from build123d import *

# Parameters (mm, degrees)
PAD011_DEPTH    = 1.2
PAD012_DEPTH    = 15.6
PAD013_DEPTH    = 1.2
PAD014_DEPTH    = 1.6
PAD015_DEPTH    = 1.6
CHAMFER004_SIZE = 1
FILLET002_R     = 1


with BuildPart() as part:
    # Sketch018 → Pad011 (new body)
    with BuildSketch(Plane.XY):
        with BuildLine():
            ThreePointArc((-94.2875364362, 7.682478298), (-94.6, 0), (-94.2875364362, -7.682478298))
            Line((-94.2875364362, -7.682478298), (-82.6504571335, -7.6824782979))
            Line((-82.6504571335, 7.682478298), (-82.6504571335, -7.6824782979))
            Line((-94.2875364362, 7.682478298), (-82.6504571335, 7.682478298))
        make_face()
    extrude(amount=PAD011_DEPTH)

    # Sketch019 → Pad012 (join)
    with BuildSketch(Plane.XY.offset(1.2)):
        with BuildLine():
            ThreePointArc((-94.2875364362, 7.682478298), (-94.6, 0), (-94.2875364362, -7.682478298))
            Line((-93.0835083525, -7.682478298), (-94.2875364362, -7.682478298))
            ThreePointArc((-93.0835083525, 7.682478298), (-93.4, 0), (-93.0835083525, -7.682478298))
            Line((-94.2875364362, 7.682478298), (-93.0835083525, 7.682478298))
        make_face()
    extrude(amount=PAD012_DEPTH)

    # Sketch020 → Pad013 (join)
    with BuildSketch(Plane.XY.offset(16.8)):
        with BuildLine():
            ThreePointArc((-94.2875364362, 7.682478298), (-94.6, 0), (-94.2875364362, -7.682478298))
            Line((-94.2875364362, -7.682478298), (-82.6504571335, -7.682478298))
            Line((-82.6504571335, 7.682478298), (-82.6504571335, -7.682478298))
            Line((-94.2875364362, 7.682478298), (-82.6504571335, 7.682478298))
        make_face()
    extrude(amount=PAD013_DEPTH)

    # Sketch021 → Pad014 (join)
    with BuildSketch(Plane.XY.offset(1.2)):
        with BuildLine():
            ThreePointArc((-84.2504571335, 7.682478298), (-84.6, 0), (-84.2504571335, -7.682478298))
            Line((-82.6504571335, -7.682478298), (-84.2504571335, -7.682478298))
            Line((-82.6504571335, 7.682478298), (-82.6504571335, -7.682478298))
            Line((-84.2504571335, 7.682478298), (-82.6504571335, 7.682478298))
        make_face()
    extrude(amount=PAD014_DEPTH)

    # Sketch022 → Pad015 (join)
    with BuildSketch(Plane.XY.offset(16.8)):
        with BuildLine():
            ThreePointArc((-84.2504571335, 7.682478298), (-84.6, 0), (-84.2504571335, -7.682478298))
            Line((-82.6504571335, -7.682478298), (-84.2504571335, -7.682478298))
            Line((-82.6504571335, 7.682478298), (-82.6504571335, -7.682478298))
            Line((-84.2504571335, 7.682478298), (-82.6504571335, 7.682478298))
        make_face()
    extrude(amount=-PAD015_DEPTH)

    # Chamfer004
    chamfer004_edges = [part.edges().sort_by_distance(p)[0] for p in [
        (-82.650457, 0, 2.8),
        (-82.650457, 0, 15.2),
    ]]
    chamfer(chamfer004_edges, length=CHAMFER004_SIZE)

    # Fillet002
    fillet002_edges = [part.edges().sort_by_distance(p)[0] for p in [
        (-94.6, 0, 18),
        (-94.6, 0, 0),
        (-82.650457, 0, 18),
        (-82.650457, 0, 0),
        (-83.950457, -7.682478, 2.8),
        (-83.950457, 7.682478, 2.8),
        (-83.950457, 7.682478, 15.2),
        (-83.950457, -7.682478, 15.2),
    ]]
    fillet(fillet002_edges, radius=FILLET002_R)


with BuildPart() as part_1:
    # Body005 placement: moved
    add(part.part.moved(Location((0, 0, -1.4))))


solid = part_1.part
Geometry: final body of the model. Coordinates: model frame, mm. A direction names the side the tool comes from. Round coordinates to 2 decimals unless told otherwise and drop trailing zeros. Loops run counter-clockwise (first coordinate to the right, second up) from the corner with the lowest first, then second, coordinate; pieces in that order, holes last. Notation, with made-up numbers: M 4.5,22.5 L 42.5,22.5 A11 ccw 42.5,40.5 Z; hole C 81.25,1.5 d6. An arc over 180 degrees is marked long. Put each result on its own line as item: value. Start each with the question number.
(1) Draft query along Z for faces 1 (the face through (-82.65, 0, 0)), 2 (the face through (-89, 0, 16.6)), 3 (the face through (-83.16, 0.11, 0.91)), 4 (the face through (-89, 0, -0.2)). Return one class per face: +Z half, -Z half, draft (parallel to the pull), parting line (faces both ways), or undercut.
(2) Contact query for flat-ended pins moving along their axis: pin 1 Ø1 at (y, z) = (4, 5.5) entering from +X; pin 2 Ø1 at (y, z) = (3.5, 4) entering from -X; pin 3 Ø2 at (y, z) = (5, 9.5) entering from -X. Output: stop coordinate, or through.
(3) Section query B-B (z = 14.25). Return loops of the section in (x, y), then the cut area to 3 significant figures.
(4) Section query C-C (z = 7.25). Return loops of the section in (x, y).
(5) Section query A-A (x = -88). Return loops of the section in (y, z), then the cut area to 3 significant figures.
(6) Material intervals for line 1 along Z through (x, y) = (-91.25, -2.5); line 2 along X through (y, z) = (0, 0); line 3 along X through (y, z) = (4, 14.5), sorted ascending. Write a range as [from, to].
(7) Set-up query: faces 5 (the face through (-93.4, 0.1, 7.5)), 6 (the face through (-84, 0, 13.8)), 7 (the face through (-83.856, 7.495, 14.217)). Return all of +Z, -Z, +X, -X, +Y, -Y with unobstructed straight access to the full face (end or side cutting, diameter ignored); none if empty.
Findings below:
1. face 1: draft
1. face 2: +Z half
1. face 3: undercut
1. face 4: undercut
2. pin 1: stops at x = -93.29
2. pin 2: stops at x = -94.55
2. pin 3: stops at x = -94.52
3. outline: M -94.29,-7.68 L -93.08,-7.68 A93.4 cw -93.08,7.68 L -94.29,7.68 A94.6 ccw Z; M -84.27,-7.52 L -83.2,-7.52 L -83.2,7.52 L -84.27,7.52 A84.6 ccw Z
3. area: 37.8 mm2
4. outline: M -94.29,-7.68 L -93.08,-7.68 A93.4 cw -93.08,7.68 L -94.29,7.68 A94.6 ccw Z
5. outline: M -7.68,-1.4 L 7.68,-1.4 L 7.68,-0.2 L -7.68,-0.2 Z; M -7.68,15.4 L 7.68,15.4 L 7.68,16.6 L -7.68,16.6 Z
5. area: 36.9 mm2
6. line 1: z = [-1.4, -0.2], [15.4, 16.6]
6. line 2: x = [-94.6, -93.4], [-84.6, -82.65]
6. line 3: x = [-94.52, -93.31], [-84.51, -82.95]
7. face 5: none
7. face 6: +X, +Y, -Y
7. face 7: +X, +Y
